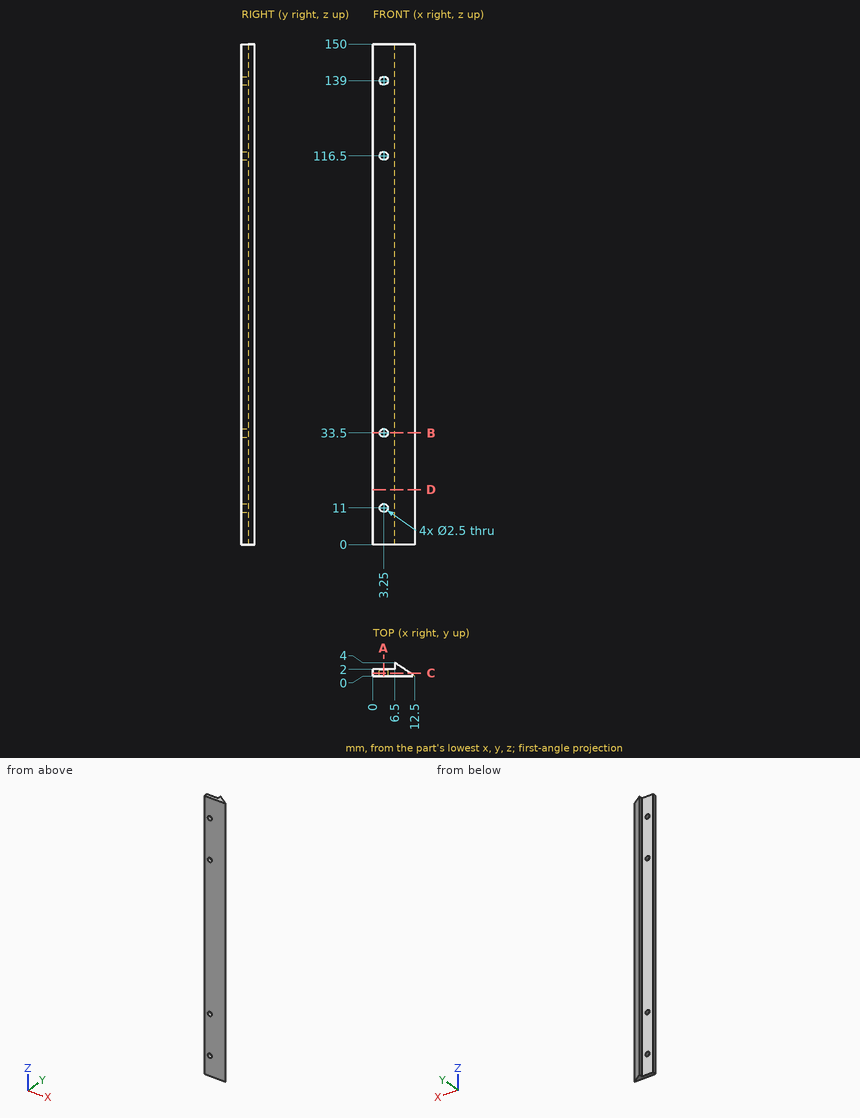
The drawing under review shows one solid part. Ordinate dimensions are in mm from its lowest x, y, z. Round coordinates to 2 decimals unless told otherwise and drop trailing zeros. Order: outer loops, then holes, each group sorted by start corner. A loop starts at its lowest first (then second) coordinate and runs counter-clockwise, first axis right, second up. Notation, with made-up numbers: (18, 12.25) -> (73, 12.25) arc R16 ccw to (73, 33.25) -> close; hole circle Ø8 at (70.25, 27.5). An arc over 180 degrees is marked (long way). Use a Markdown table: item, result.
Q1. Clearance check with flat-ended pins moving along their axes: P1, Ø3, axis at x = 3.25, z = 116.5, coming from the +Y side; P2, Ø1.6, axis at y = 3, z = 63.5, coming from the -X side; P3, Ø5, axis at x = 4.5, z = 76, coming from the +Y side; P4, Ø1.5, axis at x = 3.25, z = 11, coming from the +Y side. State where each tip first meets the part, or that it passes through.
Values:
| item | result |
|---|---|
| P1 | stops at y = 2 |
| P2 | stops at x = 6.5 |
| P3 | stops at y = 4 |
| P4 | passes through |
Q2. We need section C-C on y = 0.85. Write out the cut boundary in (x, z) (3 decimals), then the cut area to 3 significant figures.
Values:
| item | result |
|---|---|
| outline | (0, 0) -> (11.225, 0) -> (11.225, 150) -> (0, 150) -> close; hole circle Ø2.5 at (3.25, 11); hole circle Ø2.5 at (3.25, 33.5); hole circle Ø2.5 at (3.25, 116.5); hole circle Ø2.5 at (3.25, 139) |
| area | 1,660 mm^2 |
Q3. We need section D-D on z = 16.5. Write out the cut boundary in (x, y).
Values:
| item | result |
|---|---|
| outline | (0, 0) -> (12.5, 0) -> (6.5, 4) -> (6.5, 2) -> (0, 2) -> close |
Q4. We need section B-B on z = 33.5. Write out the cut boundary in (x, y), then the cut area to 3 significant figures.
Values:
| item | result |
|---|---|
| outline | (0, 0) -> (2, 0) -> (2, 2) -> (0, 2) -> close; (4.5, 0) -> (12.5, 0) -> (6.5, 4) -> (6.5, 2) -> (4.5, 2) -> close |
| area | 20.0 mm^2 |
Q5. For line 1 (Z direction, x = 3.25, y = 1.55); line 2 (Y direction, x = 3, z = 46); line 3 (X direction, y = 1.05, z = 139) (3 decimals), list the stretches that pass through material, from the lowest coordinate up.
Values:
| item | result |
|---|---|
| line 1 | z = 0 to 9.75, 12.25 to 32.25, 34.75 to 115.25, 117.75 to 137.75, 140.25 to 150 |
| line 2 | y = 0 to 2 |
| line 3 | x = 0 to 2, 4.5 to 10.925 |
Q6. We need section A-A on x = 3.25. Write out the cut boundary in (y, z).
Values:
| item | result |
|---|---|
| outline | (0, 0) -> (2, 0) -> (2, 9.75) -> (0, 9.75) -> close; (0, 12.25) -> (2, 12.25) -> (2, 32.25) -> (0, 32.25) -> close; (0, 34.75) -> (2, 34.75) -> (2, 115.25) -> (0, 115.25) -> close; (0, 117.75) -> (2, 117.75) -> (2, 137.75) -> (0, 137.75) -> close; (0, 140.25) -> (2, 140.25) -> (2, 150) -> (0, 150) -> close |
